Design review of the part built by this model. Coordinates are the model's own, in mm. A direction names the side the tool comes from. Coordinates: 2 decimals unless noted, no trailing zeros. Order: outer loops, then holes, each group sorted by start corner. A loop starts at its lowest first (then second) coordinate and runs counter-clockwise, first axis right, second up. Notation, with made-up numbers: (1.5, -29) -> (44.5, -29) arc R15 cw to (44.5, -10) -> close; hole circle Ø11 at (75, 78.5). An arc over 180 degrees is marked (long way). Use a Markdown table: item, result. Add a question column.
Q1. Add section C-C (x = -496). State the section outline as (y, z) points, then the cut area to 3 significant figures.
Q2. Insertion check: pin 1 (10 mm diameter, centred on x = -266.5, y = 0.5, fed in from +Z); pin 2 (15 mm diameter, centred on x = -560, z = 136, fed in from -Y); pin 3 (21 mm diameter, centred on y = -18, z = 95, fed in from +X). Each pin has a flat end and moves straight along its axis. Give the tip position at first contact, or say it passes through.
Q3. Add section B-B (z = 85). State the section outline as (x, y) points, then the cut area to 3 significant figures.
Q4. Wall thickness on probe 1 along X at (y, z) = (-36, 45); probe 2 along Y at (x, z) = (342.5, 52); probe 3 along Z at (x, y) = (191.5, 3.5): over which ranges is each line inside the solid? List them lowest first.
Q5. The part is to be moulded in two halves that separate along X. For faces 4 (the face through (569, -7, 112)), 5 (the face through (-531, -7, 112)), 6 (the face through (-541, -7, 112)), 7 (the face through (-8, -50, 11)), say which applies: pulls with the +X half, pulls with the -X half, needs draft (parallel to the pull), parting line crosses it, or undercut.
Q6. Machinability: for faces 1 (the face through (559, -7, 112)), 2 (the face through (-556, -15, 20)), 3 (the face through (-536.07, -25.35, 149.45)), which of the approach directions +Z, -Z, +X, -X, +Y, -Y give a long, thin tool a straight path to every point of the face, cutting with its end or side? Answer none if there is none.
Q7. Add section A-A (y = 9.5). State the section outline as (x, z) points, then the cut area to 3 significant figures.
from build123d import *

# Parameters (mm, degrees)
SKETCH_1_W             = 1142
SKETCH_1_H             = 100
EXTRUDE_1_DEPTH        = 20
SKETCH_2_W             = 1142
SKETCH_2_H             = 30
EXTRUDE_2_DEPTH        = 242
EXTRUDE_START          = -30
EXTRUDE_3_DEPTH        = 10
PATTERN_LINEAR_1_COUNT = 3
PATTERN_LINEAR_1_PITCH = 550


with BuildPart() as part:
    # Sketch 1 → Extrude 1 (new body)
    with BuildSketch(Plane.XY):
        Rectangle(SKETCH_1_W, SKETCH_1_H)
    extrude(amount=EXTRUDE_1_DEPTH)



with BuildPart() as body_2:
    # Sketch 2 → Extrude 2 (new body)
    with BuildSketch(Plane.XY.offset(20)):
        with Locations((0, 35)):
            Rectangle(SKETCH_2_W, SKETCH_2_H)
    extrude(amount=EXTRUDE_2_DEPTH)


with BuildPart() as part_1:
    add(part.part)

    add(body_2.part)  # Extrude 3 merges body 2
    # Sketch 3 → Extrude 3 (add)
    with BuildSketch(Plane.ZY.offset(571).offset(EXTRUDE_START)):
        Polygon((262, 20), (20, 20), (20, -50), (40, -50), (262, 0), align=None)
    extrude_3 = extrude(amount=-EXTRUDE_3_DEPTH)

    # Pattern Linear 1: Extrude 3 ×3
    with Locations(*[(i * PATTERN_LINEAR_1_PITCH, 0, 0) for i in range(1, PATTERN_LINEAR_1_COUNT)]):
        add(extrude_3)


solid = part_1.part
Established:
| question | item | result |
|---|---|---|
| 1 | outline | (-50, 0) -> (50, 0) -> (50, 262) -> (20, 262) -> (20, 20) -> (-50, 20) -> close |
| 1 | area | 9,260 mm^2 |
| 2 | pin 1 | z = 20 |
| 2 | pin 2 | y = 20 |
| 2 | pin 3 | x = 569 |
| 3 | outline | (-571, 20) -> (-541, 20) -> (-541, -39.86) -> (-531, -39.86) -> (-531, 20) -> (9, 20) -> (9, -39.86) -> (19, -39.86) -> (19, 20) -> (559, 20) -> (559, -39.86) -> (569, -39.86) -> (569, 20) -> (571, 20) -> (571, 50) -> (-571, 50) -> close |
| 3 | area | 36,100 mm^2 |
| 4 | probe 1 | -541 to -531, 9 to 19, 559 to 569 |
| 4 | probe 2 | 20 to 50 |
| 4 | probe 3 | 0 to 20 |
| 5 | face 4 | pulls with the +X half |
| 5 | face 5 | undercut |
| 5 | face 6 | pulls with the -X half |
| 5 | face 7 | needs draft |
| 6 | face 1 | +Z, -Y |
| 6 | face 2 | +Z, -X, -Y |
| 6 | face 3 | +Z, +X, -X, -Y |
| 7 | outline | (-571, 0) -> (571, 0) -> (571, 20) -> (569, 20) -> (569, 262) -> (559, 262) -> (559, 20) -> (19, 20) -> (19, 262) -> (9, 262) -> (9, 20) -> (-531, 20) -> (-531, 262) -> (-541, 262) -> (-541, 20) -> (-571, 20) -> close |
| 7 | area | 30,100 mm^2 |
